Could you check a few things on this model? Use its own coordinates, in mm. A direction names the side the tool comes from. Round coordinates to 2 decimals unless told otherwise and drop trailing zeros. Loops run counter-clockwise (first coordinate to the right, second up) from the corner with the lowest first, then second, coordinate; pieces in that order, holes last. Notation, with made-up numbers: (19.5, 15.25) - (32.5, 15.25) arc R26 cw to (32.5, 42.25) - close; hole circle Ø9 at (-33, 41). An arc over 180 degrees is marked (long way). Put each result on its own line as item: value. Start each with the question number.
from build123d import *

# Parameters (mm, degrees)
F0_W     = 420
F0_H     = 460
F1_DEPTH = 15
F2_R     = 3.25
F3_DEPTH = 15
F4_W     = 402
F4_H     = 402
F5_DEPTH = 5.5
F6_R     = 5.25
F7_DEPTH = 6.5
F8_DEPTH = 6.5


with BuildPart() as f1:
    # F0 (on Top) → F1 (new body)
    with BuildSketch(Plane.XY):
        with Locations((135.56531, 178.600564)):
            Rectangle(F0_W, F0_H)
    extrude(amount=F1_DEPTH)

    # F2 (on face) → F3 (cut)
    with BuildSketch(Plane.XY.offset(15)):
        with Locations((-59.43469, -41.399436)):
            Circle(F2_R)
        with Locations((-59.43469, 398.600564)):
            Circle(F2_R)
    extrude(amount=-F3_DEPTH, mode=Mode.SUBTRACT)

    # F4 (on face) → F5 (cut)
    with BuildSketch(Plane(origin=(0, 0, 0), x_dir=(1, 0, 0), z_dir=(0, 0, -1))):
        with Locations((135.56531, -178.600564)):
            Rectangle(F4_W, F4_H)
    extrude(amount=-F5_DEPTH, mode=Mode.SUBTRACT)

    # F6 (on face) → F7 (cut)
    with BuildSketch(Plane(origin=(0, 0, 0), x_dir=(1, 0, 0), z_dir=(0, 0, -1))):
        with Locations((-59.43469, -398.600564)):
            Circle(F6_R)
        with Locations((-59.43469, 41.399436)):
            Circle(F6_R)
    extrude(amount=-F7_DEPTH, mode=Mode.SUBTRACT)

    # F6 (on face) → F8 (cut)
    with BuildSketch(Plane(origin=(0, 0, 0), x_dir=(1, 0, 0), z_dir=(0, 0, -1))):
        with Locations((-59.43469, -398.600564)):
            Circle(F6_R)
        with Locations((-59.43469, 41.399436)):
            Circle(F6_R)
    extrude(amount=-F8_DEPTH, mode=Mode.SUBTRACT)


solid = f1.part
Item 1: Suppose I cut it at A-A, the plane y = 334.5. List the corners of the cut face in (x, z) for me, then the cut area to 3 significant figures.
Item 2: I need wall thicknesses on line 1 (X direction, y = 85, z = 2.25); line 2 (Y direction, x = 248.5, z = 2.5); line 3 (Z direction, x = 235, y = 238.5). Which ranges of each line are inside material? Lowest first, please. Write a range as from..to.
Item 3: Thinking about a two-plate mould opening in X: for faces 1 (the face through (-74.435, 175, 7)), 2 (the face through (133, 182, 15)), 3 (the face through (-62, -39, 6.5)), which applies, released by +X, released by -X, zero draft, split by the parting line, or undercut?
Item 4: Will these pins go through, and if not, where does the flat tip stop? P1, Ø6, axis at x = -59.43, y = 398.6, coming from the -Z side; P2, Ø17, axis at x = -59.43, y = 398.6, coming from the +Z side; P3, Ø1, axis at x = 132, y = 354.5, coming from the -Z side; P4, Ø3, axis at x = -58.5, y = -39, coming from the -Z side.
Item 5: Suppose I cut it at B-B, the plane x = 294. List the corners of the cut face in (y, z) for me, then the cut area to 3 significant figures.
Item 6: On a 3-axis mill with a long thin cutter (end or side, diameter ignored), from which of +Z, -Z, +X, -X, +Y, -Y can I reach the whole of each face in a straight line? I mean faces 4 (the face through (-57, 396, 6.5)), 5 (the face through (345.565, 175, 7)). Say none if no direction works.
Numbers:
1. outline: (-74.43, 0) - (-65.43, 0) - (-65.43, 5.5) - (336.57, 5.5) - (336.57, 0) - (345.57, 0) - (345.57, 15) - (-74.43, 15) - close
1. area: 4,090 mm^2
2. line 1: -74.43..-65.43, 336.57..345.57
2. line 2: -51.4..-22.4, 379.6..408.6
2. line 3: 5.5..15
3. face 1: released by -X
3. face 2: zero draft
3. face 3: undercut
4. P1: through
4. P2: z = 15
4. P3: z = 5.5
4. P4: z = 6.5
5. outline: (-51.4, 0) - (-22.4, 0) - (-22.4, 5.5) - (379.6, 5.5) - (379.6, 0) - (408.6, 0) - (408.6, 15) - (-51.4, 15) - close
5. area: 4,690 mm^2
6. face 4: -Z
6. face 5: +Z, -Z, +X, +Y, -Y
